Check sheet for the modelled part. Datum: model origin and axes. Units: mm. A direction names the side the tool comes from. Round coordinates to 2 decimals unless told otherwise and drop trailing zeros. Write each loop counter-clockwise with the first axis right and the second up, starting at its lowest first coordinate (ties: lowest second). Pieces come first, ordered by that corner, then holes. Notation, with made-up numbers: M 58.25,47 L 87.25,47 A7 ccw 87.25,51 Z; hole C 62,79 d3. An arc over 180 degrees is marked long. Answer in a Markdown table with one row per item.
```python
from build123d import *

# Parameters (mm, degrees)
M3_TAPPED_HOLE1_D           = 2.5
M3_TAPPED_HOLE1_DEPTH       = 7.5
M3_TAPPED_HOLE1_TIP         = 0.751075774
M5_TAPPED_HOLE1_D           = 4.2
M5_TAPPED_HOLE1_DEPTH       = 12.4
M5_TAPPED_HOLE1_CSINK_D     = 5.05
M5_TAPPED_HOLE1_CSINK_ANGLE = 90
M5_TAPPED_HOLE1_TIP         = 1.2618073


with BuildPart() as part:
    # Sketch1 → Revolve1 (revolve)
    with BuildSketch(Plane(origin=(0, 0, 0), x_dir=(1, 0, 0), z_dir=(0, 1, 0))):
        with BuildLine():
            ThreePointArc((0, -6.5), (-4.596194078, -4.596194078), (-6.5, 0))
            Line((-6.5, 0), (-18.5, 0))
            Line((-18.5, 0), (-20, -1.5))
            Line((-20, -1.5), (-20, -13.627898949))
            Line((-20, -13.627898949), (-19, -13.627898949))
            Line((-19, -13.627898949), (-19, -15.627898949))
            ThreePointArc((-19, -15.627898949), (-9.590436029, -13.660086986), (0, -13))
            Line((0, -13), (0, -6.5))
        make_face()
    revolve(axis=Axis((0, 0, -56.528501867), (0, 0, 1)))

    # M3 Tapped Hole1
    with Locations(Plane(origin=(0, 0, 0), x_dir=(-1, 0, 0), z_dir=(0, 0, -1))):
        with Locations((0, -10.795), (-9.348744234, 5.3975), (9.348744234, 5.3975)):
            Hole(M3_TAPPED_HOLE1_D / 2, depth=M3_TAPPED_HOLE1_DEPTH)
            with Locations((0, 0, -(M3_TAPPED_HOLE1_DEPTH + M3_TAPPED_HOLE1_TIP / 2))):  # 118° drill point
                Cone(0, M3_TAPPED_HOLE1_D / 2, M3_TAPPED_HOLE1_TIP, mode=Mode.SUBTRACT)

    # M5 Tapped Hole1
    with Locations(Plane(origin=(0, 20, 0), x_dir=(1, 0, 0), z_dir=(0, 1, 0))):
        with Locations((0, -5.3)):
            CounterSinkHole(M5_TAPPED_HOLE1_D / 2, M5_TAPPED_HOLE1_CSINK_D / 2, depth=M5_TAPPED_HOLE1_DEPTH, counter_sink_angle=M5_TAPPED_HOLE1_CSINK_ANGLE)
            with Locations((0, 0, -(M5_TAPPED_HOLE1_DEPTH + M5_TAPPED_HOLE1_TIP / 2))):  # 118° drill point
                Cone(0, M5_TAPPED_HOLE1_D / 2, M5_TAPPED_HOLE1_TIP, mode=Mode.SUBTRACT)


solid = part.part
```
1. Go/stop test with flat-tipped pins: pin 1 (2 mm diameter, centred on x = 9.35, y = 5.4, fed in from +Z); pin 2 (3 mm diameter, centred on x = 0, y = -10.795, fed in from +Z); pin 3 (6 mm diameter, centred on y = -8.5, z = 7, fed in from +X). Record where each tip stops, or that it passes through.
Found:
| item | result |
|---|---|
| pin 1 | stops at z = 14 |
| pin 2 | stops at z = 14.09 |
| pin 3 | stops at x = 19.23 |
2. Scan lines: L1, parallel to Y at x = -0.5, z = 4.5; L2, parallel to Y at x = -0.5, z = 10; L3, parallel to Y at x = 0, z = 2.5 (3 decimals). Record each from-to range of solid material in increasing order.
Found:
| item | result |
|---|---|
| L1 | y = -19.99 to -11.94, -9.65 to -4.66, 4.66 to 6.91 |
| L2 | y = -19.99 to 19.99 |
| L3 | y = -20 to -12.045, -9.545 to -6, 6 to 20 |
3. Section check C-C, the plane z = 14.5. Record the cut outline in (x, y).
Found:
| item | result |
|---|---|
| outline | C 0,0 d38; hole C 0,0 d28.83 |
4. Section check B-B, the plane z = 2. Count the separate pieces of the cut face and the enclosed holes in it, and give its area (3 significant figures).
Found:
| item | result |
|---|---|
| separate pieces | 1 |
| enclosed holes | 4 |
| area | 1,120 mm2 |
5. Access from +Z, -Z, +X, -X, +Y, -Y to the whole of each face (thin tool, end or side, straight path). Record for faces 4 (the face through (10.54, 5.77, 3.8)), 5 (the face through (0.273, 13.504, 3.218)), 6 (the face through (-8.767, 16.856, 14.642)).
Found:
| item | result |
|---|---|
| face 4 | -Z |
| face 5 | +Y |
| face 6 | +Z |
6. Section check A-A, the plane y = 0. Record the cut outline in (x, z), and give its area (3 significant figures).
Found:
| item | result |
|---|---|
| outline | M -20,1.5 L -18.5,0 L -6.5,0 A6.5 cw 6.5,0 L 18.5,0 L 20,1.5 L 20,13.63 L 19,13.63 L 19,15.63 A70 cw -19,15.63 L -19,13.63 L -20,13.63 Z |
| area | 486 mm2 |
7. Draft check along X on faces 1 (the face through (0.03, -10.58, 8.12)), 2 (the face through (4.336, 19.524, 7.649)), 3 (the face through (8, 0, 0)). Enter one of: +X half, -X half, draft (parallel to the pull), parting line (faces both ways), or undercut.
Found:
| item | result |
|---|---|
| face 1 | undercut |
| face 2 | parting line |
| face 3 | draft |
